Can you work these out from the model? Positions are in its coordinate system, mm. Face numbers are marked on the shaded views. Coordinates: 2 decimals unless noted, no trailing zeros. Loops run counter-clockwise (first coordinate to the right, second up) from the corner with the lowest first, then second, coordinate; pieces in that order, holes last.
```python
from build123d import *

# Parameters (mm, degrees)
F0_R     = 12
F1_DEPTH = 45
F2_R     = 6.85
F3_DEPTH = 50
F4_R     = 1.8
F5_DEPTH = 25
F6_R     = 2


with BuildPart() as f1:
    # F0 (on Front) → F1 (new body)
    with BuildSketch(Plane.XZ):
        Circle(F0_R)
    extrude(amount=F1_DEPTH)

    # F2 (on face) → F3 (cut)
    with BuildSketch(Plane.XZ.offset(45)):
        Circle(F2_R)
    extrude(amount=-F3_DEPTH, mode=Mode.SUBTRACT)

    # F4 (on Right) → F5 (cut)
    with BuildSketch(Plane.YZ):
        with Locations((-40.5, 0)):
            Circle(F4_R)
    extrude(amount=-F5_DEPTH, mode=Mode.SUBTRACT)

    # F6
    f6_edges = [f1.edges().sort_by_distance(p)[0] for p in [
        (-6.85, 0, 0),
    ]]
    fillet(f6_edges, radius=F6_R)


solid = f1.part
```
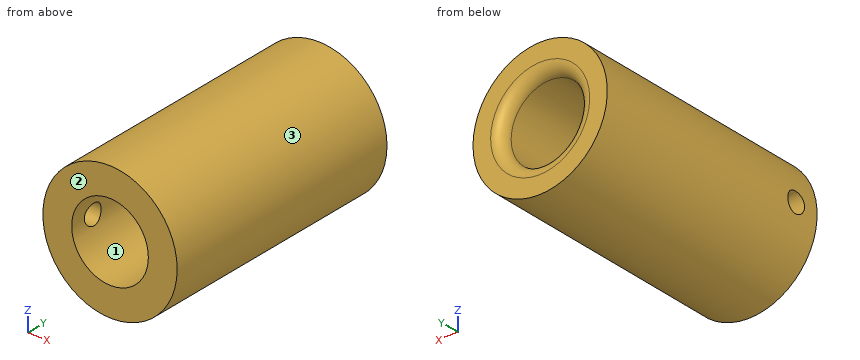
Item 1: Suppose I cut it at A-A, the plane x = 0. Please give me the cut outline in (y, z), plus the area to 3 significant figures.
Results are:
outline: (-45, -12) - (0, -12) - (0, -8.85) arc R2 ccw to (-2, -6.85) - (-45, -6.85) - close; (-45, 6.85) - (-2, 6.85) arc R2 ccw to (0, 8.85) - (0, 12) - (-45, 12) - close
area: 462 mm2
Item 2: I'm going to push flat-ended pins straight in: P1, Ø6, axis at x = -8.5, y = -22.5, coming from the -Z side; P2, Ø12, axis at x = -9, y = -38, coming from the -Z side; P3, Ø5, axis at y = -24, z = 7.5, coming from the +X side. Where does each tip first touch, or does it pass through?
Results are:
P1: stops at z = -10.67
P2: stops at z = -11.62
P3: stops at x = 10.91
Item 3: Suppose I cut it at C-C, the plane y = -16. Please give me the cut outline in (x, z).
Results are:
outline: circle Ø24 at (0, 0); hole circle Ø13.7 at (0, 0)
Item 4: Suppose I cut it at B-B, the plane z = 0. Please give me the cut outline in (x, y).
Results are:
outline: (-12, -45) - (-6.85, -45) - (-6.85, -42.3) - (-12, -42.3) - close; (-12, -38.7) - (-6.85, -38.7) - (-6.85, -2) arc R2 ccw to (-8.85, 0) - (-12, 0) - close; (6.85, -45) - (12, -45) - (12, 0) - (8.85, 0) arc R2 ccw to (6.85, -2) - close
Item 5: Suppose I cut it at D-D, the plane x = 10.25. Please give me the cut outline in (y, z).
Results are:
outline: (-45, -6.24) - (0, -6.24) - (0, 6.24) - (-45, 6.24) - close
Item 6: We'd pull the mould along X, two halves only. Please class the marked faces 1, 2 and 3: +X half, -X half, draft (parallel to the pull), parting line (faces both ways), or undercut.
Results are:
face 1: undercut
face 2: draft
face 3: parting line
Item 7: I need wall thicknesses on line 1 along X through (y, z) = (-12, 0); line 2 along Z through (x, y) = (-8.3, -40.5). Which ranges of each line are inside material? Lowest first, please.
Results are:
line 1: x = -12 to -6.85, 6.85 to 12
line 2: z = -8.67 to -1.8, 1.8 to 8.67
